from build123d import *

# Parameters (mm, degrees)
CYLINDER322_R     = 2.6
CYLINDER322_DEPTH = 10
CYLINDER321_R     = 2.6
CYLINDER321_DEPTH = 10
CYLINDER320_R     = 1.6
CYLINDER320_DEPTH = 14
CYLINDER319_R     = 1.6
CYLINDER319_DEPTH = 15
CYLINDER326_R     = 2
CYLINDER326_DEPTH = 18
CYLINDER325_R     = 2
CYLINDER325_DEPTH = 18
BOX241_W          = 69.8
BOX241_H          = 39.2
BOX241_DEPTH      = 4
BOX240_W          = 12
BOX240_H          = 30.5
BOX240_DEPTH      = 8.5
BOX235_W          = 10
BOX235_H          = 42
BOX235_DEPTH      = 10
FILLET123_R       = 2


with BuildPart() as zylinder324:
    # Cylinder322 → Cylinder322 (new body)
    with BuildSketch(Plane(origin=(-40.5, -17.5, 24), x_dir=(1, 0, 0), z_dir=(0, 0, 1))):
        Circle(CYLINDER322_R)
    extrude(amount=CYLINDER322_DEPTH)


with BuildPart() as zylinder323:
    # Cylinder321 → Cylinder321 (new body)
    with BuildSketch(Plane(origin=(-40.5, 17.5, 24), x_dir=(1, 0, 0), z_dir=(0, 0, 1))):
        Circle(CYLINDER321_R)
    extrude(amount=CYLINDER321_DEPTH)


with BuildPart() as zylinder322:
    # Cylinder320 → Cylinder320 (new body)
    with BuildSketch(Plane(origin=(-40.5, 17.5, 13), x_dir=(1, 0, 0), z_dir=(0, 0, 1))):
        Circle(CYLINDER320_R)
    extrude(amount=CYLINDER320_DEPTH)


with BuildPart() as zylinder321:
    # Cylinder319 → Cylinder319 (new body)
    with BuildSketch(Plane(origin=(-40.5, -17.5, 12.25), x_dir=(1, 0, 0), z_dir=(0, 0, 1))):
        Circle(CYLINDER319_R)
    extrude(amount=CYLINDER319_DEPTH)


with BuildPart() as zylinder328:
    # Cylinder326 → Cylinder326 (new body)
    with BuildSketch(Plane(origin=(-40.5, -2, 12.25), x_dir=(1, 0, 0), z_dir=(0, 0, 1))):
        Circle(CYLINDER326_R)
    extrude(amount=CYLINDER326_DEPTH)


with BuildPart() as fusion217:
    # Cylinder325 → Cylinder325 (new body)
    with BuildSketch(Plane(origin=(-40.5, -17.5, 12.25), x_dir=(1, 0, 0), z_dir=(0, 0, 1))):
        Circle(CYLINDER325_R)
    extrude(amount=CYLINDER325_DEPTH)

    # Fusion217: union Zylinder328
    add(zylinder328.part)


with BuildPart() as fusion217_1:
    # Fusion217 placement: moved
    add(fusion217.part.moved(Location((0, 9.75, 0))))


with BuildPart() as board006:
    # Box241 → Box241 (new body)
    with BuildSketch(Plane(origin=(-43, -19.6, 16), x_dir=(1, 0, 0), z_dir=(0, 0, 1))):
        with Locations((34.9, 19.6)):
            Rectangle(BOX241_W, BOX241_H)
    extrude(amount=BOX241_DEPTH)


with BuildPart() as fusion216:
    # Box240 → Box240 (new body)
    with BuildSketch(Plane(origin=(-46, -15.25, 17.5), x_dir=(1, 0, 0), z_dir=(0, 0, 1))):
        with Locations((6, 15.25)):
            Rectangle(BOX240_W, BOX240_H)
    extrude(amount=BOX240_DEPTH)

    # Fusion216: union Zylinder324, Zylinder323, Zylinder322, Zylinder321, Fusion217, board006
    add(zylinder324.part)
    add(zylinder323.part)
    add(zylinder322.part)
    add(zylinder321.part)
    add(fusion217_1.part)
    add(board006.part)


with BuildPart() as cut150:
    # Box235 → Box235 (new body)
    with BuildSketch(Plane(origin=(-45, -21, 17.5), x_dir=(1, 0, 0), z_dir=(0, 0, 1))):
        with Locations((5, 21)):
            Rectangle(BOX235_W, BOX235_H)
    extrude(amount=BOX235_DEPTH)

    # Fillet123
    fillet123_edges = [cut150.edges().sort_by_distance(p)[0] for p in [
        (-40, -21, 27.5),
        (-40, 21, 27.5),
    ]]
    fillet(fillet123_edges, radius=FILLET123_R)

    # Cut150: cut Fusion216
    add(fusion216.part, mode=Mode.SUBTRACT)


with BuildPart() as cut150_1:
    # Cut150 placement: moved
    add(cut150.part.moved(Location((0, 0, 0.5))))


solid = cut150_1.part
Source: CAD feature listing. Evaluate the final solid. Frame: model axes, mm. A direction names the side the tool comes from. Give positions to 0.01 mm unless a question says otherwise; leave off trailing zeros. Loops run counter-clockwise (first coordinate to the right, second up) from the corner with the lowest first, then second, coordinate; pieces in that order, holes last. Notation, with made-up numbers: (2.5, 9) -> (37.5, 9) arc R28 cw to (37.5, 36) -> close; hole circle Ø9 at (-18, 82.5). An arc over 180 degrees is marked (long way). Use a Markdown table: item, result. Add a question column.
1) Line query: line 1 along Y through (x, z) = (-40.5, 21.25); line 2 along X through (y, z) = (17.5, 25.3); line 3 along X through (y, z) = (-17.5, 22.7). Output: solid intervals per line, ascending. Write a range as [from, to].
2) Section query C-C, the plane y = -17.5. Return the cut outline in (x, z), then the cut area to 3 significant figures.
3) Reachability of faces 1 (the face through (-40, 0, 28)), 2 (the face through (-43, 17, 19)), 3 (the face through (-40, 0, 26.5)), 4 (the face through (-39.3, -19.807, 26.226)), 5 (the face through (-40, -21, 22)) from +Z, -Z, +X, -X, +Y, -Y: full face, straight path, thin tool, end or side. Return the list, or none.
4) Pull-direction query (Y, two-part tool) for faces 6 (the face through (-40.708, -15.914, 22.472)), 7 (the face through (-39.93, 20.43, 27.4)), 8 (the face through (-39.93, -20.43, 27.4)); classes: +Y half, -Y half, draft (parallel to the pull), parting line (faces both ways), or undercut.
5) Section query A-A, the plane z = 21.25. Return the cut outline in (x, y), then the cut area to 3 significant figures.
6) Section query D-D, the plane x = -41.25. Count the separate pieces of the cut face and the enclosed holes in it, then the cut area to 3 significant figures.
7) Section query B-B, the plane y = 7.75. Return the cut outline in (x, z), then the cut area to 3 significant figures.
8) First-contact query: pin 1 (2.5 mm diameter, centred on x = -40.5, y = -17.5, fed in from +Z); pin 2 (1.5 mm diameter, centred on x = -39, y = 3, fed in from -Z); pin 3 (2 mm diameter, centred on y = 17.5, z = 19, fed in from +X); pin 4 (2 mm diameter, centred on x = -38, y = 17.5, fed in from -Z). Flat tips, straight axial feed; report the tip coordinate or a pass-through.
Numbers:
| question | item | result |
|---|---|---|
| 1 | line 1 | y = [-21, -19.1], [-15.9, -15.25], [15.25, 15.9], [19.1, 21] |
| 1 | line 2 | x = [-45, -43.1], [-37.9, -35] |
| 1 | line 3 | x = [-45, -42.1], [-38.9, -35] |
| 2 | outline | (-45, 18) -> (-43, 18) -> (-43, 20.5) -> (-42.1, 20.5) -> (-42.1, 24.5) -> (-43.1, 24.5) -> (-43.1, 28) -> (-45, 28) -> close; (-38.9, 20.5) -> (-35, 20.5) -> (-35, 28) -> (-37.9, 28) -> (-37.9, 24.5) -> (-38.9, 24.5) -> close |
| 2 | area | 49.0 mm2 |
| 3 | face 1 | +Z, +X, -X, +Y, -Y |
| 3 | face 2 | -Z, +X |
| 3 | face 3 | -Z, +X, -X |
| 3 | face 4 | +Z |
| 3 | face 5 | +Z, -Z, +X, -X, -Y |
| 4 | face 6 | undercut |
| 4 | face 7 | +Y half |
| 4 | face 8 | -Y half |
| 5 | outline | (-45, -21) -> (-35, -21) -> (-35, -15.25) -> (-45, -15.25) -> close; (-45, 15.25) -> (-35, 15.25) -> (-35, 21) -> (-45, 21) -> close; hole circle Ø3.2 at (-40.5, -17.5); hole circle Ø3.2 at (-40.5, 17.5) |
| 5 | area | 98.9 mm2 |
| 6 | separate pieces | 7 |
| 6 | enclosed holes | 0 |
| 6 | area | 69.8 mm2 |
| 7 | outline | (-45, 26.5) -> (-42.5, 26.5) -> (-42.5, 28) -> (-45, 28) -> close; (-38.5, 26.5) -> (-35, 26.5) -> (-35, 28) -> (-38.5, 28) -> close |
| 7 | area | 9.00 mm2 |
| 8 | pin 1 | passes through |
| 8 | pin 2 | stops at z = 26.5 |
| 8 | pin 3 | stops at x = -43 |
| 8 | pin 4 | stops at z = 20.5 |
